```python
from build123d import *

# Parameters (mm, degrees)
ESQUISSE1_W        = 175
ESQUISSE1_H        = 100
ESQUISSE1_R        = 6.25
BOSS_EXTRU_1_DEPTH = 10
CONG_1_R           = 12


with BuildPart() as part:
    # Esquisse1 → Boss.-Extru.1 (new body)
    with BuildSketch(Plane.XY):
        Rectangle(ESQUISSE1_W, ESQUISSE1_H)
        with Locations((0, 30)):
            Circle(ESQUISSE1_R, mode=Mode.SUBTRACT)
        with Locations((0, -30)):
            Circle(ESQUISSE1_R, mode=Mode.SUBTRACT)
    extrude(amount=BOSS_EXTRU_1_DEPTH)

    # Congé1
    cong_1_edges = [part.edges().sort_by_distance(p)[0] for p in [
        (87.5, -50, 5),
        (-87.5, -50, 5),
        (-87.5, 50, 5),
        (87.5, 50, 5),
    ]]
    fillet(cong_1_edges, radius=CONG_1_R)


solid = part.part
```
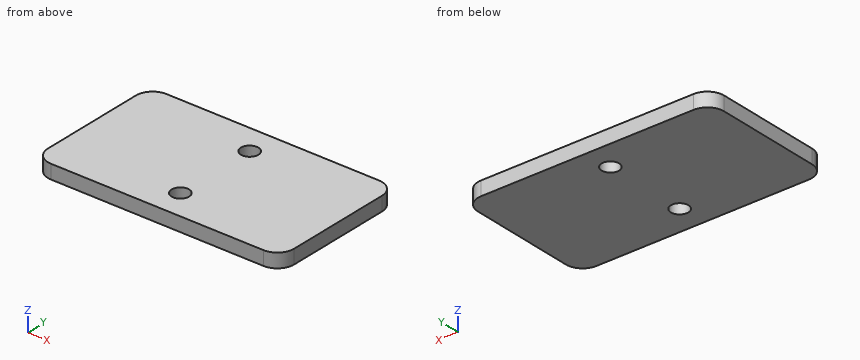
The listing builds one solid part. Answer for the finished solid, in the listing's coordinates (mm). Give positions to 0.01 mm unless a question says otherwise; leave off trailing zeros. Order: outer loops, then holes, each group sorted by start corner. A loop starts at its lowest first (then second) coordinate and runs counter-clockwise, first axis right, second up. Notation, with made-up numbers: (-2, 12) - (56, 12) arc R19 cw to (56, 43) - close; hole circle Ø2 at (71.5, 48). An arc over 180 degrees is marked (long way). Answer in a Markdown table with one row per item. Add a question column.
Q1. The part is cut by section C-C (x = 0). Determine the outline of the cut face in (y, z).
Q2. The part is cut by section A-A (y = -30). Determine the outline of the cut face in (x, z).
Q3. The part is cut by section B-B (z = 1.75). Determine the outline of the cut face in (x, y), then the cut area to 3 significant figures.
Q4. Given P1, Ø10, axis at x = 0, y = -30, coming from the -Z side, flat-ended and moving along its own axis, determine where the tip first touches the part or whether it passes through.
Q5. Find the intervals of material crossed by line 1 along Y through (x, z) = (0, 7); line 2 along X through (y, z) = (-26.5, 6.25); line 3 along X through (y, z) = (34.5, 0.75), in increasing order. Write a range as [from, to].
Determined:
| question | item | result |
|---|---|---|
| 1 | outline | (-50, 0) - (-36.25, 0) - (-36.25, 10) - (-50, 10) - close; (-23.75, 0) - (23.75, 0) - (23.75, 10) - (-23.75, 10) - close; (36.25, 0) - (50, 0) - (50, 10) - (36.25, 10) - close |
| 2 | outline | (-87.5, 0) - (-6.25, 0) - (-6.25, 10) - (-87.5, 10) - close; (6.25, 0) - (87.5, 0) - (87.5, 10) - (6.25, 10) - close |
| 3 | outline | (-87.5, -38) arc R12 ccw to (-75.5, -50) - (75.5, -50) arc R12 ccw to (87.5, -38) - (87.5, 38) arc R12 ccw to (75.5, 50) - (-75.5, 50) arc R12 ccw to (-87.5, 38) - close; hole circle Ø12.5 at (0, -30); hole circle Ø12.5 at (0, 30) |
| 3 | area | 17,100 mm² |
| 4 | P1 | passes through |
| 5 | line 1 | y = [-50, -36.25], [-23.75, 23.75], [36.25, 50] |
| 5 | line 2 | x = [-87.5, -5.18], [5.18, 87.5] |
| 5 | line 3 | x = [-87.5, -4.34], [4.34, 87.5] |
